Autodesk Inventor part; units mm, degrees
ref_plane "YZ Plane" through (0, 0, 0) normal (1, 0, 0) x (0, 1, 0)
ref_plane "XZ Plane" through (0, 0, 0) normal (0, 1, 0) x (-1, 0, 0)
ref_plane "XY Plane" through (0, 0, 0) normal (0, 0, 1) x (1, 0, 0)
sketch "Sketch1" plane through (0, 0, 0) normal (0, 0, 1) x (1, 0, 0)
  arc A0 (235.6827, -57.867) -> (240.6827, -52.867) centre (235.6827, -52.867) ccw
  line L0 (240.6827, -52.867) -> (240.6827, 24.133)
  arc A1 (240.6827, 24.133) -> (235.6827, 29.133) centre (235.6827, 24.133) ccw
  line L1 (235.6827, 29.133) -> (-24.3173, 29.133)
  arc A2 (-24.3173, 29.133) -> (-29.3173, 24.133) centre (-24.3173, 24.133) ccw
  line L2 (-29.3173, 24.133) -> (-29.3173, -52.867)
  arc A3 (-29.3173, -52.867) -> (-24.3173, -57.867) centre (-24.3173, -52.867) ccw
  line L3 (-24.3173, -57.867) -> (235.6827, -57.867)
  circle A4 centre (235.6827, 23.633) radius 1.7
  circle A5 centre (235.6827, -5.867) radius 1.7
  circle A6 centre (-24.3173, -5.867) radius 1.7
  circle A7 centre (-24.3173, 23.633) radius 1.7
  circle A8 centre (208.6827, 8.133) radius 2.75
  circle A9 centre (228.1827, -46.867) radius 3.3
  circle A10 centre (189.1827, -46.867) radius 3.3
  circle A11 centre (22.1827, -46.867) radius 3.3
  circle A12 centre (-16.8173, -46.867) radius 3.3
  circle A13 centre (235.6827, -5.867) radius 1.7
  circle A14 centre (235.6827, 23.633) radius 1.7
  circle A15 centre (-24.3173, 23.633) radius 1.7
  circle A16 centre (-24.3173, -5.867) radius 1.7
  arc A17 (235.6827, -57.867) -> (240.6827, -52.867) centre (235.6827, -52.867) ccw
  line L4 (240.6827, -52.867) -> (240.6827, 24.133)
  arc A18 (240.6827, 24.133) -> (235.6827, 29.133) centre (235.6827, 24.133) ccw
  line L5 (235.6827, 29.133) -> (172.1827, 29.133)
  arc A19 (-24.3173, 29.133) -> (-29.3173, 24.133) centre (-24.3173, 24.133) ccw
  line L6 (-29.3173, 24.133) -> (-29.3173, -52.867)
  arc A20 (-29.3173, -52.867) -> (-24.3173, -57.867) centre (-24.3173, -52.867) ccw
  line L7 (-24.3173, -57.867) -> (235.6827, -57.867)
  circle A21 centre (17.1827, -7.367) radius 3.3
  circle A22 centre (17.1827, 23.633) radius 3.3
  circle A23 centre (-13.8173, 23.633) radius 3.3
  circle A24 centre (-13.8173, -7.367) radius 3.3
  circle A25 centre (208.6827, 8.133) radius 2.75
  circle A26 centre (1.6827, 8.133) radius 11.5
  line L8 (221.1827, -40.867) -> (221.1827, -52.867)
  line L9 (221.1827, -52.867) -> (196.1827, -52.867)
  line L10 (196.1827, -52.867) -> (196.1827, -40.867)
  line L11 (196.1827, -40.867) -> (221.1827, -40.867)
  line L12 (-11.8173, -52.867) -> (-11.8173, -40.867)
  line L13 (-11.8173, -40.867) -> (15.1827, -40.867)
  line L14 (15.1827, -40.867) -> (15.1827, -52.867)
  line L15 (15.1827, -52.867) -> (-11.8173, -52.867)
  circle A27 centre (27.6827, -5.867) radius 1.7
  circle A28 centre (27.6827, 23.633) radius 1.7
  line L16 (172.1827, 29.133) -> (172.1827, -4.0741)
  line L17 (172.1827, -4.0741) -> (168.3898, -7.867)
  line L18 (168.3898, -7.867) -> (132.9756, -7.867)
  line L19 (132.9756, -7.867) -> (129.1827, -4.0741)
  line L20 (129.1827, -4.0741) -> (129.1827, 29.133)
  line L21 (129.1827, 29.133) -> (-24.3173, 29.133)
  circle A29 centre (183.6827, -5.867) radius 1.7
  circle A30 centre (183.6827, 23.633) radius 1.7
extrude "Extrusion1" add sketch "Sketch1" along normal blind 4 contours L3 A3 L2 A2 L1 L20 L19 L18 L17 L16 A1 L0 A0 | L16 L17 L18 L19 L20 L1 | A4 | A5 | A6 | A7 | A8 | A9 | A10 | A11 | A12 | A21 | A22 | A23 | A24 | A26 | A27 | A28 | A29 | A30
hole "Hole1" at (-24.3173, -5.867, 0) at (-24.3173, 23.633, 0) at (235.6827, 23.633, 0) at (235.6827, -5.867, 0) at (27.6827, 23.633, 0) at (27.6827, -5.867, 0) direction (0, 0, 1) diameter 3.4 end through all
hole "Hole2" at (208.6827, 8.133, 0) direction (0, 0, 1) diameter 5.5 end through all
hole "Hole3" at (-16.8173, -46.867, 0) at (22.1827, -46.867, 0) at (189.1827, -46.867, 0) at (228.1827, -46.867, 0) direction (0, 0, 1) diameter 3.4 end through all countersink diameter 6.6 countersink angle 90
sketch "Sketch2" plane through (0, 0, 4) normal (0, 0, 1) x (1, 0, 0)
  circle A0 centre (166.1827, -1.867) radius 1.7
  circle A1 centre (166.1827, 29.133) radius 1.7
  circle A2 centre (135.1827, 29.133) radius 1.7
  circle A3 centre (135.1827, -1.867) radius 1.7
  circle A4 centre (150.6827, 13.633) radius 11
  line L0 (168.1827, 34.633) -> (171.6827, 31.133)
  line L1 (168.1827, 34.633) -> (133.1827, 34.633)
  line L2 (129.6827, 31.133) -> (133.1827, 34.633)
  line L3 (129.6827, 31.133) -> (129.6827, -3.867)
  line L4 (133.1827, -7.367) -> (129.6827, -3.867)
  line L5 (133.1827, -7.367) -> (168.1827, -7.367)
  line L6 (171.6827, -3.867) -> (168.1827, -7.367)
  line L7 (171.6827, -3.867) -> (171.6827, 31.133)
  circle A5 centre (150.6827, 13.633) radius 11.5
  line L8 (150.6827, -7.367) -> (150.6827, -57.867)
  line L9 (-24.3173, -57.867) -> (235.6827, -57.867)
  line L10 (150.6827, -32.617) -> (163.331, -32.617) construction
  circle A6 centre (183.6827, 23.633) radius 1.7
  circle A7 centre (183.6827, -5.867) radius 1.7
  point P0 (0, 0)
  point P1 (150.6827, -17.367)
  point P2 (150.6827, -47.867)
  dimension "d23" = 0.5
  dimension "d35" = 10
extrude "Extrusion2" cut sketch "Sketch2" against normal through all contours A4 | A5
sketch "Sketch3" plane through (0, 0, 4) normal (0, 0, 1) x (1, 0, 0)
  circle A0 centre (166.1827, -1.867) radius 1.7
  circle A1 centre (166.1827, 29.133) radius 1.7
  circle A2 centre (135.1827, 29.133) radius 1.7
  circle A3 centre (135.1827, -1.867) radius 1.7
  circle A4 centre (150.6827, 13.633) radius 11
  line L0 (168.1827, 34.633) -> (171.6827, 31.133)
  line L1 (168.1827, 34.633) -> (133.1827, 34.633)
  line L2 (129.6827, 31.133) -> (133.1827, 34.633)
  line L3 (129.6827, 31.133) -> (129.6827, -3.867)
  line L4 (133.1827, -7.367) -> (129.6827, -3.867)
  line L5 (133.1827, -7.367) -> (168.1827, -7.367)
  line L6 (171.6827, -3.867) -> (168.1827, -7.367)
  line L7 (171.6827, -3.867) -> (171.6827, 31.133)
  line L8 (235.6827, 29.133) -> (-24.3173, 29.133)
  point P0 (0, 0)
  point P1 (129.6827, 29.133)
  point P2 (171.6827, 29.133)
extrude "Extrusion3" add sketch "Sketch3" against normal blind 4 contours L8 A1 | A1 L8 A2 L3 L2 L1 L0 L7 | L8 A2 picked at (166.251, 30.4471) picked at (135.251, 30.4471)
hole "Hole4" at (135.1827, -1.867, 4) at (135.1827, 29.133, 4) at (166.1827, 29.133, 4) at (166.1827, -1.867, 4) direction (0, 0, -1) diameter 3.4 end through all countersink diameter 6.6 countersink angle 90
sketch "Sketch4" plane through (0, 0, 0) normal (0, 0, -1) x (-1, 0, 0)
  point P0 (0, 0)
  point P1 (-150.6827, -17.367)
  point P2 (-150.6827, -47.867)
hole "Hole5" at (150.6827, -17.367, 0) at (150.6827, -47.867, 0) direction (0, 0, 1) diameter 4.3 end through all countersink diameter 8.6 countersink angle 90
hole "Hole6" at (183.6827, 23.633, 4) at (183.6827, -5.867, 4) direction (0, 0, -1) diameter 3.4 end through all countersink diameter 6.6 countersink angle 90
properties part number "plate_2"
Verification items for the finished model (mm, model axes). Round coordinates to 2 decimals unless told otherwise and drop trailing zeros. Write each loop counter-clockwise with the first axis right and the second up, starting at its lowest first coordinate (ties: lowest second). Pieces come first, ordered by that corner, then holes.
(1) Section check B-B (y = 16). Enter the section's corners in (x, z).
Returned:
outline: (-29.32, 0) - (139.43, 0) - (139.43, 4) - (-29.32, 4) - close; (161.94, 0) - (240.68, 0) - (240.68, 4) - (161.94, 4) - close
(2) Depth check by flat-ended pin: pin 1 Ø1.6 at (y, z) = (30.5, 1.5) entering from +X; pin 2 Ø4 at (x, y) = (189.18, -46.87) entering from -Z; pin 3 Ø2 at (x, z) = (212.5, 1.5) entering from +Y. Enter the tip coordinate at first touch or a pass-through.
Returned:
pin 1: stops at x = 171.68
pin 2: stops at z = 1.3
pin 3: stops at y = 29.13
(3) Mould release check, pull along Y, two halves, no side actions. Record for faces 1 (the flat face through (104, -11, 4)), 2 (the cylindrical face through (-27.814, -56.441, 1.972)), 3 (the cylindrical face through (205.956, 7.775, 2.028)): pulls with the +Y half, pulls with the -Y half, needs draft (parallel to the pull), parting line crosses it, or undercut.
Returned:
face 1: needs draft
face 2: pulls with the -Y half
face 3: undercut
(4) Section check A-A (x = 214). Enter the section's corners in (y, z), plus the area to 3 significant figures.
Returned:
outline: (-57.87, 0) - (-52.87, 0) - (-52.87, 4) - (-57.87, 4) - close; (-40.87, 0) - (29.13, 0) - (29.13, 4) - (-40.87, 4) - close
area: 300 mm2
(5) Section check C-C (x = 47). Enter the section's corners in (y, z), plus the area to 3 significant figures.
Returned:
outline: (-57.87, 0) - (29.13, 0) - (29.13, 4) - (-57.87, 4) - close
area: 348 mm2
(6) Material ranges on line 1 (X direction, y = -43, z = 2.15); line 2 (Y direction, x = 15, z = 2.45); line 3 (X direction, y = -1.5, z = 2.3), recorded low to high.
Returned:
line 1: x = -29.32 to -11.82, 15.18 to 196.18, 221.18 to 240.68
line 2: y = -57.87 to -52.87, -40.87 to 29.13
line 3: x = -29.32 to 133.52, 136.84 to 164.52, 167.84 to 240.68
